Read the model definition and answer for the solid it produces. Units are mm, in the model's axes. A direction names the side the tool comes from. Coordinates: 2 decimals unless noted, no trailing zeros. Loops run counter-clockwise (first coordinate to the right, second up) from the corner with the lowest first, then second, coordinate; pieces in that order, holes last.
from build123d import *
from OCP.BRepFilletAPI import BRepFilletAPI_MakeFillet

# Parameters (mm, degrees)
SKETCH_1_W          = 38
SKETCH_1_H          = 33
EXTRUDE_1_DEPTH     = 2
SKETCH_2_R          = 2.025
CUT_EXTRUDE_1_DEPTH = 2
SKETCH_3_W          = 50
SKETCH_3_H          = 16
CUT_EXTRUDE_2_DEPTH = 2
FILLET_1_R1         = 2
FILLET_1_R2         = 4
SKETCH_4_W          = 5
SKETCH_4_H          = 33
CUT_EXTRUDE_3_DEPTH = 2
CHAMFER_1_SIZE      = 10
FILLET_2_R          = 2


with BuildPart() as part:
    # Sketch 1 → Extrude 1 (new body)
    with BuildSketch(Plane.XY):
        Rectangle(SKETCH_1_W, SKETCH_1_H)
    extrude(amount=EXTRUDE_1_DEPTH)

    # Sketch 2 → Cut-Extrude 1 (cut)
    with BuildSketch(Plane.XY.offset(2)):
        with Locations((-10, 0)):
            Circle(SKETCH_2_R)
        with Locations((15, -12)):
            Circle(SKETCH_2_R)
        with Locations((15, 12)):
            Circle(SKETCH_2_R)
    extrude(amount=-CUT_EXTRUDE_1_DEPTH, mode=Mode.SUBTRACT)

    # Sketch 3 → Cut-Extrude 2 (cut)
    with BuildSketch(Plane.XY.offset(2)):
        with Locations((19, 0)):
            Rectangle(SKETCH_3_W, SKETCH_3_H)
    extrude(amount=-CUT_EXTRUDE_2_DEPTH, mode=Mode.SUBTRACT)

    # Fillet 1: one fillet with a radius per group of edges: ONE call of the kernel's fillet builder (fillet() takes one radius for all edges)
    fillet_1_edges_1 = [part.edges().sort_by_distance(p)[0] for p in [
        (-6, -8, 1),
        (-6, 8, 1),
        (19, -16.5, 1),
        (19, 16.5, 1),
    ]]
    fillet_1_edges_2 = [part.edges().sort_by_distance(p)[0] for p in [
        (19, 8, 1),
        (19, -8, 1),
    ]]
    fillet_1 = BRepFilletAPI_MakeFillet(part.part.solid().wrapped)
    for e in fillet_1_edges_1:
        fillet_1.Add(FILLET_1_R1, e.wrapped)
    for e in fillet_1_edges_2:
        fillet_1.Add(FILLET_1_R2, e.wrapped)
    add(Compound.cast(fillet_1.Shape()), mode=Mode.REPLACE)

    # Sketch 4 → Cut-Extrude 3 (cut)
    with BuildSketch(Plane.XY.offset(2)):
        with Locations((-16.5, 0)):
            Rectangle(SKETCH_4_W, SKETCH_4_H)
    extrude(amount=-CUT_EXTRUDE_3_DEPTH, mode=Mode.SUBTRACT)

    # Chamfer 1
    chamfer_1_edges = [part.edges().sort_by_distance(p)[0] for p in [
        (-14, 16.5, 1),
        (-14, -16.5, 1),
    ]]
    chamfer(chamfer_1_edges, length=CHAMFER_1_SIZE)

    # Fillet 2
    fillet_2_edges = [part.edges().sort_by_distance(p)[0] for p in [
        (-4, 16.5, 1),
        (-14, -6.5, 1),
        (-14, 6.5, 1),
        (-4, -16.5, 1),
    ]]
    fillet(fillet_2_edges, radius=FILLET_2_R)


solid = part.part
Item 1: A cutting plane is placed at C-C on z = 0.95. Determine the outline of the cut face in (x, y) (3 decimals).
Numbers:
outline: (-14, -5.672) arc R2 ccw to (-13.414, -7.086) - (-4.586, -15.914) arc R2 ccw to (-3.172, -16.5) - (17, -16.5) arc R2 ccw to (19, -14.5) - (19, -12) arc R4 ccw to (15, -8) - (-4, -8) arc R2 cw to (-6, -6) - (-6, 6) arc R2 cw to (-4, 8) - (15, 8) arc R4 ccw to (19, 12) - (19, 14.5) arc R2 ccw to (17, 16.5) - (-3.172, 16.5) arc R2 ccw to (-4.586, 15.914) - (-13.414, 7.086) arc R2 ccw to (-14, 5.672) - close; hole circle Ø4.05 at (-10, 0); hole circle Ø4.05 at (15, -12); hole circle Ø4.05 at (15, 12)
Item 2: A cutting plane is placed at B-B on y = 0. Determine the outline of the cut face in (x, z) (3 decimals).
Numbers:
outline: (-14, 0) - (-12.025, 0) - (-12.025, 2) - (-14, 2) - close; (-7.975, 0) - (-6, 0) - (-6, 2) - (-7.975, 2) - close
Item 3: Determine the mould class of faces 1 (the face through (16.87, -12.78, 1.01)), 2 (the face through (19, -13, 1)), 3 (the face through (-9.1, -11.4, 1)) for opening direction X: released by +X, released by -X, zero draft, split by the parting line, or undercut.
Numbers:
face 1: undercut
face 2: released by +X
face 3: released by -X
Item 4: A cutting plane is placed at D-D on x = 13.5. Determine the outline of the cut face in (y, z), then the cut area to 3 significant figures.
Numbers:
outline: (-16.5, 0) - (-13.36, 0) - (-13.36, 2) - (-16.5, 2) - close; (-10.64, 0) - (-8, 0) - (-8, 2) - (-10.64, 2) - close; (8, 0) - (10.64, 0) - (10.64, 2) - (8, 2) - close; (13.36, 0) - (16.5, 0) - (16.5, 2) - (13.36, 2) - close
area: 23.1 mm2
Item 5: Find the intervals of material crossed by line 1 along Y through (x, z) = (15, 0.7) (3 decimals); line 2 along Y through (x, z) = (10.5, 0.9); line 3 along Y through (x, z) = (-10, 1.4) (3 decimals), in increasing order.
Numbers:
line 1: y = -16.5 to -14.025, -9.975 to -8, 8 to 9.975, 14.025 to 16.5
line 2: y = -16.5 to -8, 8 to 16.5
line 3: y = -10.5 to -2.025, 2.025 to 10.5
Item 6: A cutting plane is placed at A-A on x = -10. Determine the outline of the cut face in (y, z) (3 decimals), then the cut area to 3 significant figures.
Numbers:
outline: (-10.5, 0) - (-2.025, 0) - (-2.025, 2) - (-10.5, 2) - close; (2.025, 0) - (10.5, 0) - (10.5, 2) - (2.025, 2) - close
area: 33.9 mm2
Item 7: Which of the six approach directions +Z, -Z, +X, -X, +Y, -Y give full straight-line access (tool end or side, diameter ignored) to faces 4 (the face through (-14, 0, 1)), 5 (the face through (17.859, -9.203, 1.014))?
Numbers:
face 4: +Z, -Z, -X, +Y, -Y
face 5: +Z, -Z, +X
Item 8: Given pin 1 (0.6 mm diameter, centred on y = 2, z = 1, fed in from +X), flat-ended and moving along its own axis, determine where the tip first touches the part or whether it passes through.
Numbers:
pin 1: stops at x = -6
